```python
from build123d import *

# Parameters (mm, degrees)
SKETCH3_W           = 220
SKETCH3_H           = 280
BOSS_EXTRUDE1_DEPTH = 3.175
SKETCH4_W           = 10
SKETCH4_H           = 10
BOSS_EXTRUDE2_DEPTH = 50
SKETCH7_R           = 2
SKETCH7_R_2         = 2.000000006
SKETCH7_R_3         = 1.999999994
CUT_EXTRUDE2_DEPTH  = 10
CUT_EXTRUDE4_DEPTH  = 10


with BuildPart() as part:
    # Sketch3 → Boss-Extrude1 (new body)
    with BuildSketch(Plane(origin=(0, 0, 0), x_dir=(1, 0, 0), z_dir=(0, 1, 0))):
        Rectangle(SKETCH3_W, SKETCH3_H)
    extrude(amount=BOSS_EXTRUDE1_DEPTH)

    # Sketch4 → Boss-Extrude2 (add)
    with BuildSketch(Plane(origin=(0, 3.175, 0), x_dir=(1, 0, 0), z_dir=(0, 1, 0))):
        with Locations((105, -135)):
            Rectangle(SKETCH4_W, SKETCH4_H)
        with Locations((105, -70)):
            Rectangle(SKETCH4_W, SKETCH4_H)
        with Locations((40, -135)):
            Rectangle(SKETCH4_W, SKETCH4_H)
        with Locations((40, -70)):
            Rectangle(SKETCH4_W, SKETCH4_H)
    extrude(amount=BOSS_EXTRUDE2_DEPTH)

    # Sketch7 → Cut-Extrude2 (cut)
    with BuildSketch(Plane.XZ):
        with Locations(Location((-103, 70, 0), (0, 0, 270))):
            Circle(SKETCH7_R)
        with Locations(Location((-103, 110, 0), (0, 0, 270))):
            Circle(SKETCH7_R)
        with Locations(Location((-85, 110, 0), (0, 0, 270))):
            Circle(SKETCH7_R_2)
        with Locations(Location((-85, 70, 0), (0, 0, 270))):
            Circle(SKETCH7_R)
        with Locations(Location((85, 110, 0), (0, 0, 270))):
            Circle(SKETCH7_R_3)
        with Locations(Location((103, 110, 0), (0, 0, 270))):
            Circle(SKETCH7_R)
        with Locations(Location((103, 70, 0), (0, 0, 270))):
            Circle(SKETCH7_R)
        with Locations(Location((85, 70, 0), (0, 0, 270))):
            Circle(SKETCH7_R)
        with Locations(Location((106, -107, 0), (0, 0, 270))):
            Circle(SKETCH7_R)
        with Locations(Location((84, -85, 0), (0, 0, 270))):
            Circle(SKETCH7_R)
        with Locations(Location((106, -85, 0), (0, 0, 270))):
            Circle(SKETCH7_R)
        with Locations(Location((84, -107, 0), (0, 0, 270))):
            Circle(SKETCH7_R)
        with Locations(Location((-84, -107, 0), (0, 0, 270))):
            Circle(SKETCH7_R)
        with Locations(Location((-106, -107, 0), (0, 0, 270))):
            Circle(SKETCH7_R)
        with Locations(Location((-106, -85, 0), (0, 0, 270))):
            Circle(SKETCH7_R)
        with Locations(Location((-84, -85, 0), (0, 0, 270))):
            Circle(SKETCH7_R)
    extrude(amount=-CUT_EXTRUDE2_DEPTH, mode=Mode.SUBTRACT)

    # Sketch9 → Cut-Extrude4 (cut)
    with BuildSketch(Plane(origin=(0, 3.175, 0), x_dir=(1, 0, 0), z_dir=(0, 1, 0))):
        Polygon((0, 70), (75, 140), (-75, 140), align=None)
    extrude(amount=-CUT_EXTRUDE4_DEPTH, mode=Mode.SUBTRACT)


solid = part.part
```
Geometry: final body of the model. Coordinates: model frame, mm. A direction names the side the tool comes from. Coordinates: 2 decimals unless noted, no trailing zeros. Order: outer loops, then holes, each group sorted by start corner. A loop starts at its lowest first (then second) coordinate and runs counter-clockwise, first axis right, second up. Notation, with made-up numbers: (-11, 67.5) -> (25, 67.5) arc R18 ccw to (25, 87.5) -> close; hole circle Ø10 at (-4, 34.5). An arc over 180 degrees is marked (long way). Write item = value, one per line.
(1) Cut plane A-A on y = 16.5. Return loops of the section in (x, z).
Solved:
outline = (35, 65) -> (45, 65) -> (45, 75) -> (35, 75) -> close; (35, 130) -> (45, 130) -> (45, 140) -> (35, 140) -> close; (100, 65) -> (110, 65) -> (110, 75) -> (100, 75) -> close; (100, 130) -> (110, 130) -> (110, 140) -> (100, 140) -> close
(2) Cut plane D-D on z = 49. Return loops of the section in (x, y) (3 decimals).
Solved:
outline = (-110, 0) -> (110, 0) -> (110, 3.175) -> (-110, 3.175) -> close
(3) Access query for faces 1 (the flat face through (45, 28, 135)), 2 (the flat face through (105, 28, 75)), 3 (the flat face through (35, 28, 70)), 4 (the flat face through (36.975, 1.61, -104.51)), 5 (the flat face through (40, 28, 65)). Directions: +Z, -Z, +X, -X, +Y, -Y. A direction counts if a zero-diameter tool reaches every point of the face in a straight line with its end or side. Return the directions, or none.
Solved:
face_1 = +Z, -Z, +Y
face_2 = +X, -X, +Y
face_3 = +Z, -Z, -X, +Y
face_4 = -Z, +Y, -Y
face_5 = -Z, +X, -X, +Y
(4) Cut plane C-C on x = 93. Return loops of the section in (y, z) (3 decimals).
Solved:
outline = (0, -140) -> (3.175, -140) -> (3.175, 140) -> (0, 140) -> close
(5) Line query: line 1 (X direction, y = 2.3, z = 110); line 2 (X direction, y = 2.45, z = -107); line 3 (Z direction, x = 40, y = 29). Output: solid intervals per line, ascending.
Solved:
line_1 = -110 to -105, -101 to -87, -83 to 83, 87 to 101, 105 to 110
line_2 = -110 to -108, -104 to -86, -82 to -39.64, 39.64 to 82, 86 to 104, 108 to 110
line_3 = 65 to 75, 130 to 140
(6) Pull-direction query (X, two-part tool) for faces 6 (the flat face through (105, 28, 130)), 7 (the flat face through (-38.025, 1.61, -105.49)), 8 (the flat face through (110, 1, 53)); classes: pulls with the +X half, pulls with the -X half, needs draft (parallel to the pull), parting line crosses it, or undercut.
Solved:
face_6 = needs draft
face_7 = undercut
face_8 = pulls with the +X half
(7) Pin query (flat end, axial travel): pin 1 Ø2 at (x, z) = (0.5, -25.5) entering from +Y (3 decimals); pin 2 Ø5 at (x, y) = (40, 35) entering from -Z; pin 3 Ø3 at (y, z) = (35, 69.5) entering from -X. Return the tip coordinate at first contact, or that it passes through.
Solved:
pin_1 = 3.175
pin_2 = 65
pin_3 = 35
(8) Cut plane B-B on z = -76.5. Return loops of the section in (x, y) (3 decimals).
Solved:
outline = (-110, 0) -> (-6.964, 0) -> (-6.964, 3.175) -> (-110, 3.175) -> close; (6.964, 0) -> (110, 0) -> (110, 3.175) -> (6.964, 3.175) -> close
